from build123d import *

# Parameters (mm, degrees)
SKETCH1_R           = 1.65
SKETCH1_R_2         = 2
BOSS_EXTRUDE1_DEPTH = 3.175
SKETCH2_W           = 3.175
SKETCH2_H           = 8
CUT_EXTRUDE1_DEPTH  = 4.175


with BuildPart() as part:
    # Sketch1 → Boss-Extrude1 (new body)
    with BuildSketch(Plane(origin=(0, 0, 0), x_dir=(-1, 0, 0), z_dir=(0, 0, 1))):
        with BuildLine():
            Line((0, -62.136729163), (0, 62.869580678))
            ThreePointArc((0, 62.869580678), (-48.575, 0.366425758), (0, -62.136729163))
        make_face()
        with Locations((-5.075, 56.366425758)):
            Circle(SKETCH1_R, mode=Mode.SUBTRACT)
        with Locations((-21.638471196, 46.366425758)):
            Circle(SKETCH1_R, mode=Mode.SUBTRACT)
        with Locations((-5.075, -55.633574242)):
            Circle(SKETCH1_R, mode=Mode.SUBTRACT)
        with Locations((-21.638471196, -45.633574242)):
            Circle(SKETCH1_R, mode=Mode.SUBTRACT)
        with Locations((-38, 20.287222228)):
            Circle(SKETCH1_R_2, mode=Mode.SUBTRACT)
        with Locations((-38.301731617, -19.711639731)):
            Circle(SKETCH1_R_2, mode=Mode.SUBTRACT)
    extrude(amount=BOSS_EXTRUDE1_DEPTH)

    # Sketch2 → Cut-Extrude1 (cut, through all)
    with BuildSketch(Plane.XY.offset(3.175)):
        with Locations((32.4875, 9.633574242)):
            Rectangle(SKETCH2_W, SKETCH2_H)
        with Locations((32.4875, -10.366425758)):
            Rectangle(SKETCH2_W, SKETCH2_H)
    extrude(amount=-CUT_EXTRUDE1_DEPTH, mode=Mode.SUBTRACT)


solid = part.part
Geometry: final body of the model. Coordinates: model frame, mm. A direction names the side the tool comes from. Give positions to 0.01 mm unless a question says otherwise; leave off trailing zeros. Write each loop counter-clockwise with the first axis right and the second up, starting at its lowest first coordinate (ties: lowest second). Pieces come first, ordered by that corner, then holes. Notation, with made-up numbers: M -25,-27 L 27,-27 A29 cw 27,12 Z; hole C 37,29.25 d6. An arc over 180 degrees is marked long. Answer in a Markdown table with one row per item. Add a question column.
(1) Section D-D on y = -29. Return loops of the section in (x, z) (3 decimals), and give its area (3 significant figures).
(2) First-contact query: pin 1 (1.6 mm diameter, centred on x = 33, z = 1, fed in from -Y); pin 2 (1.6 mm diameter, centred on x = 32.5, z = 1.5, fed in from +Y). Flat tips, straight axial feed; report the tip coordinate or a pass-through.
(3) Reachability of faces 4 (the flat face through (32, -14.366, 2)), 5 (the flat face through (19, -1, 0)) from +Z, -Z, +X, -X, +Y, -Y: full face, straight path, thin tool, end or side. Return the list, or none.
(4) Mould query, pull axis X, two halves, no side actions, for faces 1 (the flat face through (19, -1, 3.175)), 2 (the flat face through (0, 1, 2)), 3 (the flat face through (34.075, 10, 2)). Classes: +X half, -X half, draft (parallel to the pull), parting line (faces both ways), or undercut.
(5) Section B-B on z = 2.1. State how many separate pieces and enclosed holes the cut face has, and give its area (3 significant figures).
(6) Ray query, line 1 (Y direction, x = 38, z = 1.2); line 2 (X direction, y = -8, z = 1.55) (3 decimals); line 3 (X direction, y = -13.5, z = 2.8) (3 decimals). Return the intervals inside material, ascending.
(7) Section A-A on x = 38. Return loops of the section in (y, z) (3 decimals), and give its area (3 significant figures).
(8) Section C-C on y = -51. Return loops of the section in (x, z) (3 decimals).
Result set:
| question | item | result |
|---|---|---|
| 1 | outline | M 0,0 L 41.871,0 L 41.871,3.175 L 0,3.175 Z |
| 1 | area | 133 mm^2 |
| 2 | pin 1 | stops at y = -43.31 |
| 2 | pin 2 | stops at y = 43.13 |
| 3 | face 4 | +Z, -Z |
| 3 | face 5 | -Z, +X, -X, +Y, -Y |
| 4 | face 1 | draft |
| 4 | face 2 | -X half |
| 4 | face 3 | undercut |
| 5 | separate pieces | 1 |
| 5 | enclosed holes | 8 |
| 5 | area | 4,390 mm^2 |
| 6 | line 1 | y = -35.75 to -22.29, -18.29 to 17.73, 21.69 to 35.02 |
| 6 | line 2 | x = 0 to 30.9, 34.075 to 48.122 |
| 6 | line 3 | x = 0 to 30.9, 34.075 to 47.224 |
| 7 | outline | M -35.755,0 L -22.287,0 L -22.287,3.175 L -35.755,3.175 Z; M -18.287,0 L 17.735,0 L 17.735,3.175 L -18.287,3.175 Z; M 21.689,0 L 35.022,0 L 35.022,3.175 L 21.689,3.175 Z |
| 7 | area | 199 mm^2 |
| 8 | outline | M 0,0 L 24.031,0 L 24.031,3.175 L 0,3.175 Z |
